```python
from build123d import *

# Parameters (mm, degrees)
ESBO_O1_W                = 120
ESBO_O1_H                = 97
RESSALTO_EXTRUS_O1_DEPTH = 3
ESBO_O2_W                = 16
ESBO_O2_H                = 15
CORTE_EXTRUS_O1_DEPTH    = 78.209131584
PADR_O_LINEAR1_COUNT     = 2
PADR_O_LINEAR1_PITCH     = 20


with BuildPart() as part:
    # Esboço1 → Ressalto-extrusão1 (new body)
    with BuildSketch(Plane.XY):
        Rectangle(ESBO_O1_W, ESBO_O1_H)
    extrude(amount=RESSALTO_EXTRUS_O1_DEPTH)

    # Esboço2 → Corte-extrusão1 (cut, through all)
    with BuildSketch(Plane.XY.offset(3)):
        with Locations((-1.5, -31)):
            Rectangle(ESBO_O2_W, ESBO_O2_H)
    corte_extrus_o1 = extrude(amount=-CORTE_EXTRUS_O1_DEPTH, mode=Mode.SUBTRACT)

    # Padrão linear1: Corte-extrusão1 ×2
    with Locations(*[(0, i * PADR_O_LINEAR1_PITCH, 0) for i in range(1, PADR_O_LINEAR1_COUNT)]):
        add(corte_extrus_o1, mode=Mode.SUBTRACT)


solid = part.part
```
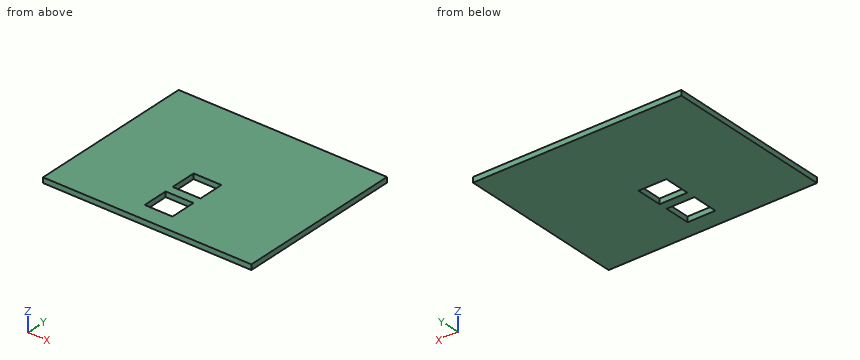
Input: part model. Units: mm. Frame: model coordinates. Coordinates: 2 decimals unless noted, no trailing zeros. Order: outer loops, then holes, each group sorted by start corner. A loop starts at its lowest first (then second) coordinate and runs counter-clockwise, first axis right, second up. Notation, with made-up numbers: (-35.5, -37.5) - (9.5, -37.5) arc R30 cw to (9.5, -6.5) - close; hole circle Ø1 at (28, 82). An arc over 180 degrees is marked (long way). Put each result on its own line as item: value.
1. Cut plane B-B on z = 2.3. Return the cut outline in (x, y), then the cut area to 3 significant figures.
Report:
outline: (-60, -48.5) - (60, -48.5) - (60, 48.5) - (-60, 48.5) - close; hole (-9.5, -38.5) - (6.5, -38.5) - (6.5, -23.5) - (-9.5, -23.5) - close; hole (-9.5, -18.5) - (6.5, -18.5) - (6.5, -3.5) - (-9.5, -3.5) - close
area: 11,200 mm2
2. Line query: line 1 along Y through (x, z) = (-1, 1.4); line 2 along X through (y, z) = (-31.5, 1.4). Output: solid intervals per line, ascending.
Report:
line 1: y = -48.5 to -38.5, -23.5 to -18.5, -3.5 to 48.5
line 2: x = -60 to -9.5, 6.5 to 60
3. Cut plane A-A on y = -11. Return the cut outline in (x, z), then the cut area to 3 significant figures.
Report:
outline: (-60, 0) - (-9.5, 0) - (-9.5, 3) - (-60, 3) - close; (6.5, 0) - (60, 0) - (60, 3) - (6.5, 3) - close
area: 312 mm2
